Geometry check sheet. Reference: the model listing, model coordinates, mm. Round coordinates to 2 decimals unless told otherwise and drop trailing zeros. Loops run counter-clockwise (first coordinate to the right, second up) from the corner with the lowest first, then second, coordinate; pieces in that order, holes last. Notation, with made-up numbers: M 70.25,33.25 L 118.25,33.25 A20 cw 118.25,47.25 Z; hole C 80.25,-33.75 d8. An arc over 180 degrees is marked long. Use one line per item in the form item = value. Start each with the question number.
1. Material ranges on line 1 (Z direction, x = 124.9, y = 1.4); line 2 (Z direction, x = 225, y = 1.25); line 3 (Z direction, x = 51.5, y = 4.3), recorded low to high.
2. Cross-section at A-A (x = 105). Record the boundary of the cut face in (y, z).
3. Go/stop test with a flat-tipped pin: pin 1 (3 mm diameter, centred on x = 91.5, z = -64, fed in from -Y). Record where the tip stops, or that it passes through.
4. Cross-section at B-B (z = -190). Record the boundary of the cut face in (x, y), then the cut area to 3 significant figures.
5. Cross-section at C-C (z = -120.5). Record the boundary of the cut face in (x, y).
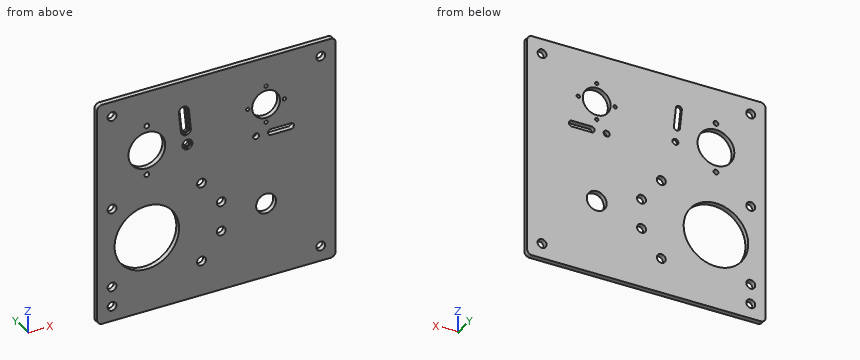
```python
from build123d import *

# Parameters (mm, degrees)
SKETCH1_W            = 230
SKETCH1_H            = 200
BOSS_EXTRUDE1_DEPTH  = 5
SKETCH2_R            = 18.5
SKETCH2_R_2          = 14
SKETCH2_R_3          = 10
SKETCH2_R_4          = 15
SKETCH2_R_5          = 3
CUT_EXTRUDE1_DEPTH   = 305.836021494
M3_CLEARANCE_HOLE1_D = 3.4
SKETCH6_R            = 3
CUT_EXTRUDE3_DEPTH   = 305.836021494
SKETCH7_R            = 32.5
CUT_EXTRUDE4_DEPTH   = 305.836021494
SKETCH8_W            = 10
SKETCH8_H            = 200
BOSS_EXTRUDE2_DEPTH  = 5
SKETCH9_W            = 240
SKETCH9_H            = 25
BOSS_EXTRUDE3_DEPTH  = 5
M8_CLEARANCE_HOLE1_D = 9
FILLET2_R            = 5
M8_CLEARANCE_HOLE2_D = 9
M8_CLEARANCE_HOLE3_D = 9
SKETCH21_R           = 5
CUT_EXTRUDE5_DEPTH   = 2.5
SKETCH22_R           = 2.4
CUT_EXTRUDE6_DEPTH   = 330.013677527


with BuildPart() as part:
    # Sketch1 → Boss-Extrude1 (new body)
    with BuildSketch(Plane(origin=(0, 0, 0), x_dir=(1, 0, 0), z_dir=(0, 1, 0))):
        with Locations((115, 100)):
            Rectangle(SKETCH1_W, SKETCH1_H)
    extrude(amount=BOSS_EXTRUDE1_DEPTH)

    # Sketch2 → Cut-Extrude1 (cut, through all)
    with BuildSketch(Plane(origin=(0, 5, 0), x_dir=(1, 0, 0), z_dir=(0, 1, 0))):
        with Locations(Location((50, 60, 0), (0, 0, 270))):
            Circle(SKETCH2_R)
        with Locations(Location((169.999156247, 48, 0), (0, 0, 270))):
            Circle(SKETCH2_R_2)
        with Locations(Location((169.999156247, 150, 0), (0, 0, 90))):
            Circle(SKETCH2_R_3)
        with Locations(Location((50, 149.55, 0), (0, 0, 90))):
            Circle(SKETCH2_R_4)
        with Locations(Location((90.796528955, 65.97019474, 0), (0, 0, 270))):
            Circle(SKETCH2_R_5)
        with BuildLine():
            Line((92.289074142, 50.746124691), (90.298985907, 30.845382272))
            ThreePointArc((90.298985907, 30.845382272), (87.015361309, 28.158784144), (84.328763181, 31.442408742))
            Line((84.328763181, 31.442408742), (86.318851416, 51.343151161))
            ThreePointArc((86.318851416, 51.343151161), (89.602476014, 54.029749289), (92.289074142, 50.746124691))
        make_face()
    extrude(amount=-CUT_EXTRUDE1_DEPTH, mode=Mode.SUBTRACT)

    # M3 Clearance Hole1 (through all)
    with Locations(Plane(origin=(0, 5, 0), x_dir=(1, 0, 0), z_dir=(0, 1, 0))):
        with Locations((151.499156247, 48), (50, 35), (50, 85), (169.999156247, 66.5), (169.999156247, 29.5), (188.499156247, 48)):
            Hole(M3_CLEARANCE_HOLE1_D / 2)

    # Sketch6 → Cut-Extrude3 (cut, through all)
    with BuildSketch(Plane(origin=(0, 5, 0), x_dir=(1, 0, 0), z_dir=(0, 1, 0))):
        with Locations(Location((159.999156247, 78, 0), (0, 0, 270))):
            Circle(SKETCH6_R)
        with BuildLine():
            Line((174.999156247, 81), (194.999156247, 81))
            ThreePointArc((194.999156247, 81), (197.999156247, 78), (194.999156247, 75))
            Line((194.999156247, 75), (174.999156247, 75))
            ThreePointArc((174.999156247, 75), (171.999156247, 78), (174.999156247, 81))
        make_face()
    extrude(amount=-CUT_EXTRUDE3_DEPTH, mode=Mode.SUBTRACT)

    # Sketch7 → Cut-Extrude4 (cut, through all)
    with BuildSketch(Plane(origin=(0, 5, 0), x_dir=(1, 0, 0), z_dir=(0, 1, 0))):
        with Locations(Location((50, 149.55, 0), (0, 0, 270))):
            Circle(SKETCH7_R)
    extrude(amount=-CUT_EXTRUDE4_DEPTH, mode=Mode.SUBTRACT)

    # Sketch8 → Boss-Extrude2 (add)
    with BuildSketch(Plane(origin=(0, 5, 0), x_dir=(1, 0, 0), z_dir=(0, 1, 0))):
        with Locations((235, 100)):
            Rectangle(SKETCH8_W, SKETCH8_H)
    extrude(amount=-BOSS_EXTRUDE2_DEPTH)

    # Sketch9 → Boss-Extrude3 (add)
    with BuildSketch(Plane(origin=(0, 5, 0), x_dir=(1, 0, 0), z_dir=(0, 1, 0))):
        with Locations((120, 212.5)):
            Rectangle(SKETCH9_W, SKETCH9_H)
    extrude(amount=-BOSS_EXTRUDE3_DEPTH)

    # M8 Clearance Hole1 (through all)
    with Locations(Plane(origin=(0, 5, 0), x_dir=(1, 0, 0), z_dir=(0, 1, 0))):
        with Locations((15, 210), (225, 210), (225, 15), (15, 15)):
            Hole(M8_CLEARANCE_HOLE1_D / 2)

    # Fillet2
    fillet2_edges = [part.edges().sort_by_distance(p)[0] for p in [
        (240, 2.5, 0),
        (240, 2.5, -225),
        (0, 2.5, -225),
        (0, 2.5, 0),
    ]]
    fillet(fillet2_edges, radius=FILLET2_R)

    # M8 Clearance Hole2 (through all)
    with Locations(Plane(origin=(0, 0, 0), x_dir=(-1, 0, 0), z_dir=(0, -1, 0))):
        with Locations((-15, 190), (-105, 190), (-105, 110), (-15, 110)):
            Hole(M8_CLEARANCE_HOLE2_D / 2)

    # M8 Clearance Hole3 (through all)
    with Locations(Plane(origin=(0, 5, 0), x_dir=(1, 0, 0), z_dir=(0, 1, 0))):
        with Locations((124.9, 165), (124.9, 135)):
            Hole(M8_CLEARANCE_HOLE3_D / 2)

    # Sketch21 → Cut-Extrude5 (cut)
    with BuildSketch(Plane.XZ):
        with Locations(Location((90.796528955, -65.97019474, 0), (0, 0, 270))):
            Circle(SKETCH21_R)
        with BuildLine():
            Line((82.338688939, -31.641417566), (84.328777174, -51.542159985))
            ThreePointArc((84.328777174, -51.542159985), (89.801484838, -56.019823531), (94.279148384, -50.547115867))
            Line((94.279148384, -50.547115867), (92.289060149, -30.646373448))
            ThreePointArc((92.289060149, -30.646373448), (86.816352485, -26.168709902), (82.338688939, -31.641417566))
        make_face()
    extrude(amount=-CUT_EXTRUDE5_DEPTH, mode=Mode.SUBTRACT)

    # Sketch22 → Cut-Extrude6 (cut, through all)
    with BuildSketch(Plane(origin=(0, 5, 0), x_dir=(1, 0, 0), z_dir=(0, 1, 0))):
        with Locations(Location((50, 85, 0), (0, 0, 270))):
            Circle(SKETCH22_R)
        with Locations(Location((50, 35, 0), (0, 0, 270))):
            Circle(SKETCH22_R)
    extrude(amount=-CUT_EXTRUDE6_DEPTH, mode=Mode.SUBTRACT)


solid = part.part
```
Reported:
q1.line_1 = -225 to -169.5, -160.5 to -139.5, -130.5 to 0
q1.line_2 = -225 to -214.5, -205.5 to -19.5, -10.5 to 0
q1.line_3 = -225 to -182.02, -117.08 to -86.87, -83.13 to -78.44, -41.56 to -36.87, -33.13 to 0
q2.outline = M 0,-225 L 5,-225 L 5,-194.5 L 0,-194.5 Z; M 0,-185.5 L 5,-185.5 L 5,-114.5 L 0,-114.5 Z; M 0,-105.5 L 5,-105.5 L 5,0 L 0,0 Z
q3.pin_1 = 2.5
q4.outline = M 0,0 L 10.5,0 L 10.5,5 L 0,5 Z; M 19.5,0 L 100.5,0 L 100.5,5 L 19.5,5 Z; M 109.5,0 L 240,0 L 240,5 L 109.5,5 Z
q4.area = 1,110 mm²
q5.outline = M 0,0 L 35.43,0 L 35.43,5 L 0,5 Z; M 64.57,0 L 240,0 L 240,5 L 64.57,5 Z
